Geometry check sheet. Reference: the model listing, model coordinates, mm. A direction names the side the tool comes from. Round coordinates to 2 decimals unless told otherwise and drop trailing zeros. Write each loop counter-clockwise with the first axis right and the second up, starting at its lowest first coordinate (ties: lowest second). Pieces come first, ordered by that corner, then holes. Notation, with made-up numbers: M 87,-8.5 L 111,-8.5 A13 ccw 111,-0.5 Z; hole C 14.5,3.5 d10. An arc over 180 degrees is marked long. Answer in a Markdown table with one row per item. Add a question column.
Autodesk Inventor part; units mm, degrees
ref_plane "YZ Plane" through (0, 0, 0) normal (1, 0, 0) x (0, 1, 0)
ref_plane "XZ Plane" through (0, 0, 0) normal (0, 1, 0) x (-1, 0, 0)
ref_plane "XY Plane" through (0, 0, 0) normal (0, 0, 1) x (1, 0, 0)
sketch "Sketch1" plane through (0, 0, 0) normal (0, 1, 0) x (-1, 0, 0)
  line L0 (-25, -25) -> (25, -25)
  line L1 (25, -25) -> (25, 25)
  line L2 (25, 25) -> (-25, 25)
  line L3 (-25, 25) -> (-25, -25)
  line L4 (-25, -25) -> (25, 25) construction
  line L5 (25, -25) -> (-25, 25) construction
  circle A0 centre (0, 0) radius 2.5
  line L6 (-22.5, -22.5) -> (-27.5, -22.5)
  line L7 (-27.5, -22.5) -> (-27.5, -27.5)
  line L8 (-27.5, -27.5) -> (-22.5, -27.5)
  line L9 (-22.5, -27.5) -> (-22.5, -22.5)
  line L10 (-22.5, -22.5) -> (-27.5, -27.5) construction
  line L11 (-27.5, -22.5) -> (-22.5, -27.5) construction
  line L12 (27.5, -22.5) -> (22.5, -22.5)
  line L13 (22.5, -22.5) -> (22.5, -27.5)
  line L14 (22.5, -27.5) -> (27.5, -27.5)
  line L15 (27.5, -27.5) -> (27.5, -22.5)
  line L16 (27.5, -22.5) -> (22.5, -27.5) construction
  line L17 (22.5, -22.5) -> (27.5, -27.5) construction
  line L18 (27.5, 27.5) -> (22.5, 27.5)
  line L19 (22.5, 27.5) -> (22.5, 22.5)
  line L20 (22.5, 22.5) -> (27.5, 22.5)
  line L21 (27.5, 22.5) -> (27.5, 27.5)
  line L22 (27.5, 27.5) -> (22.5, 22.5) construction
  line L23 (22.5, 27.5) -> (27.5, 22.5) construction
  line L24 (-22.5, 27.5) -> (-27.5, 27.5)
  line L25 (-27.5, 27.5) -> (-27.5, 22.5)
  line L26 (-27.5, 22.5) -> (-22.5, 22.5)
  line L27 (-22.5, 22.5) -> (-22.5, 27.5)
  line L28 (-22.5, 27.5) -> (-27.5, 22.5) construction
  line L29 (-27.5, 27.5) -> (-22.5, 22.5) construction
  circle A1 centre (5, -5) radius 1
  circle A2 centre (5, 5) radius 1
  circle A3 centre (-5, 5) radius 1
  circle A4 centre (-5, -5) radius 1
  point P0 (25, -22.5)
  point P1 (22.5, -25)
  point P2 (-22.5, -25)
  point P3 (-25, -22.5)
  point P4 (-25, 22.5)
  point P5 (-22.5, 25)
  point P6 (22.5, 25)
  point P7 (25, 22.5)
  point P8 (0, -25)
  point P9 (25, 0)
  point P10 (0, 25)
  point P11 (-25, 0)
  dimension "d0" = 50
  dimension "d1" = 50
  dimension "d45" = 5
  dimension "d46" = 5
  dimension "d47" = 5
  dimension "d48" = 5
  dimension "d49" = 5
  dimension "d50" = 5
  dimension "d51" = 5
  dimension "d52" = 5
  dimension "d53" = 5
  dimension "d82" = 2
  dimension "d83" = 2
  dimension "d84" = 2
  dimension "d85" = 2
  dimension "d86" = 5
  dimension "d87" = 5
  dimension "d88" = 5
  dimension "d89" = 5
  dimension "d90" = 5
  dimension "d91" = 5
  dimension "d92" = 5
  dimension "d93" = 5
extrude "Extrusion1" add sketch "Sketch1" along normal blind 5
sketch "Sketch2" plane through (0, 5, 0) normal (0, 1, 0) x (1, 0, 0)
  line L0 (-25, 22.5) -> (-25, -22.5)
  line L1 (-22.5, -25) -> (22.5, -25)
  line L2 (25, -22.5) -> (25, 22.5)
  line L3 (22.5, 25) -> (-22.5, 25)
  line L4 (25, -12.5) -> (20, -12.5)
  line L5 (20, -12.5) -> (20, -7.5)
  line L6 (20, -7.5) -> (25, -7.5)
  line L7 (25, -7.5) -> (25, -12.5)
  line L8 (25, -22.5) -> (25, 22.5)
  line L9 (25, 7.5) -> (20, 7.5)
  line L10 (20, 7.5) -> (20, 12.5)
  line L11 (20, 12.5) -> (25, 12.5)
  line L12 (25, 12.5) -> (25, 7.5)
  line L13 (-25, -12.5) -> (-20, -12.5)
  line L14 (-20, -12.5) -> (-20, -7.5)
  line L15 (-20, -7.5) -> (-25, -7.5)
  line L16 (-25, -7.5) -> (-25, -12.5)
  line L17 (-25, 22.5) -> (-25, -22.5)
  line L18 (-25, 7.5) -> (-20, 7.5)
  line L19 (-20, 7.5) -> (-20, 12.5)
  line L20 (-20, 12.5) -> (-25, 12.5)
  line L21 (-25, 12.5) -> (-25, 7.5)
  line L22 (-22.5, -25) -> (22.5, -25)
  line L23 (-25, 12.5) -> (-20, 12.5)
  line L24 (-20, 12.5) -> (-20, 13.5)
  line L25 (-20, 13.5) -> (-25, 13.5)
  line L26 (-25, 13.5) -> (-25, 12.5)
  line L27 (20, 12.5) -> (25, 12.5)
  line L28 (25, 12.5) -> (25, 13.5)
  line L29 (25, 13.5) -> (20, 13.5)
  line L30 (20, 13.5) -> (20, 12.5)
  line L31 (25, 7.5) -> (20, 7.5)
  line L32 (20, 7.5) -> (20, 6.5)
  line L33 (20, 6.5) -> (25, 6.5)
  line L34 (25, 6.5) -> (25, 7.5)
  line L35 (-20, 7.5) -> (-25, 7.5)
  line L36 (-25, 7.5) -> (-25, 6.5)
  line L37 (-25, 6.5) -> (-20, 6.5)
  line L38 (-20, 6.5) -> (-20, 7.5)
  line L39 (-25, -7.5) -> (-20, -7.5)
  line L40 (-20, -7.5) -> (-20, -6.5)
  line L41 (-20, -6.5) -> (-25, -6.5)
  line L42 (-25, -6.5) -> (-25, -7.5)
  line L43 (-25, -12.5) -> (-20, -12.5)
  line L44 (-20, -12.5) -> (-20, -13.5)
  line L45 (-20, -13.5) -> (-25, -13.5)
  line L46 (-25, -13.5) -> (-25, -12.5)
  line L47 (25, -7.5) -> (20, -7.5)
  line L48 (20, -7.5) -> (20, -6.5)
  line L49 (20, -6.5) -> (25, -6.5)
  line L50 (25, -6.5) -> (25, -7.5)
  line L51 (20, -12.5) -> (25, -12.5)
  line L52 (25, -12.5) -> (25, -13.5)
  line L53 (25, -13.5) -> (20, -13.5)
  line L54 (20, -13.5) -> (20, -12.5)
  line L55 (-25, -22.5) -> (-27.5, -22.5)
  line L56 (-27.5, -22.5) -> (-27.5, -27.5)
  line L57 (-27.5, -27.5) -> (-22.5, -27.5)
  line L58 (-22.5, -27.5) -> (-22.5, -25)
  line L59 (22.5, -25) -> (22.5, -27.5)
  line L60 (22.5, -27.5) -> (27.5, -27.5)
  line L61 (27.5, -27.5) -> (27.5, -22.5)
  line L62 (27.5, -22.5) -> (25, -22.5)
  line L63 (25, 22.5) -> (27.5, 22.5)
  line L64 (27.5, 22.5) -> (27.5, 27.5)
  line L65 (27.5, 27.5) -> (22.5, 27.5)
  line L66 (22.5, 27.5) -> (22.5, 25)
  line L67 (-22.5, 25) -> (-22.5, 27.5)
  line L68 (-22.5, 27.5) -> (-27.5, 27.5)
  line L69 (-27.5, 27.5) -> (-27.5, 22.5)
  line L70 (-27.5, 22.5) -> (-25, 22.5)
  line L71 (-12.5, 25) -> (-7.5, 25)
  line L72 (-7.5, 25) -> (-7.5, 20)
  line L73 (-7.5, 20) -> (-12.5, 20)
  line L74 (-12.5, 20) -> (-12.5, 25)
  line L75 (7.5, 25) -> (12.5, 25)
  line L76 (12.5, 25) -> (12.5, 20)
  line L77 (12.5, 20) -> (7.5, 20)
  line L78 (7.5, 20) -> (7.5, 25)
  line L79 (-12.5, -25) -> (-7.5, -25)
  line L80 (-7.5, -25) -> (-7.5, -20)
  line L81 (-7.5, -20) -> (-12.5, -20)
  line L82 (-12.5, -20) -> (-12.5, -25)
  line L83 (7.5, -25) -> (12.5, -25)
  line L84 (12.5, -25) -> (12.5, -20)
  line L85 (12.5, -20) -> (7.5, -20)
  line L86 (7.5, -20) -> (7.5, -25)
  line L87 (22.5, 25) -> (-22.5, 25)
  line L88 (-12.5, -20) -> (-13.5, -20)
  line L89 (-13.5, -20) -> (-13.5, -25)
  line L90 (-13.5, -25) -> (-12.5, -25)
  line L91 (-12.5, -25) -> (-12.5, -20)
  line L92 (-7.5, -20) -> (-6.5, -20)
  line L93 (-6.5, -20) -> (-6.5, -25)
  line L94 (-6.5, -25) -> (-7.5, -25)
  line L95 (-7.5, -25) -> (-7.5, -20)
  line L96 (7.5, -20) -> (6.5, -20)
  line L97 (6.5, -20) -> (6.5, -25)
  line L98 (6.5, -25) -> (7.5, -25)
  line L99 (7.5, -25) -> (7.5, -20)
  line L100 (12.5, -20) -> (13.5, -20)
  line L101 (13.5, -20) -> (13.5, -25)
  line L102 (13.5, -25) -> (12.5, -25)
  line L103 (12.5, -25) -> (12.5, -20)
  line L104 (-7.5, 25) -> (-6.5, 25)
  line L105 (-6.5, 25) -> (-6.5, 20)
  line L106 (-6.5, 20) -> (-7.5, 20)
  line L107 (-7.5, 20) -> (-7.5, 25)
  line L108 (7.5, 25) -> (6.5, 25)
  line L109 (6.5, 25) -> (6.5, 20)
  line L110 (6.5, 20) -> (7.5, 20)
  line L111 (7.5, 20) -> (7.5, 25)
  line L112 (12.5, 25) -> (13.5, 25)
  line L113 (13.5, 25) -> (13.5, 20)
  line L114 (13.5, 20) -> (12.5, 20)
  line L115 (12.5, 20) -> (12.5, 25)
  line L116 (-12.5, 25) -> (-13.5, 25)
  line L117 (-13.5, 25) -> (-13.5, 20)
  line L118 (-13.5, 20) -> (-12.5, 20)
  line L119 (-12.5, 20) -> (-12.5, 25)
  point P0 (0, 0)
  point P1 (-25, 25)
  point P2 (-25, -25)
  point P3 (25, -25)
  point P4 (25, 25)
  point P5 (20, -10)
  point P6 (20, 10)
  point P7 (-25, 10)
  point P8 (-25, -10)
  point P9 (-25, 6.5)
  point P10 (-25, 13.5)
  point P11 (25, 13.5)
  point P12 (25, 6.5)
  point P13 (25, -13.5)
  point P14 (-25, -13.5)
  point P15 (25, 10)
  point P16 (-25, 0)
  point P17 (0, -25)
  point P18 (-10, -25)
  point P19 (10, -25)
  point P20 (0, 25)
  point P21 (10, 25)
  point P22 (-10, 25)
  point P23 (0, 25)
  dimension "d9" = 5
  dimension "d10" = 5
  dimension "d11" = 5
  dimension "d12" = 5
  dimension "d13" = 5
  dimension "d14" = 5
  dimension "d15" = 5
  dimension "d16" = 5
  dimension "d21" = 5
  dimension "d22" = 1
  dimension "d23" = 5
  dimension "d24" = 1
  dimension "d25" = 5
  dimension "d26" = 1
  dimension "d27" = 5
  dimension "d28" = 1
  dimension "d29" = 5
  dimension "d30" = 1
  dimension "d31" = 5
  dimension "d32" = 1
  dimension "d33" = 5
  dimension "d34" = 1
  dimension "d35" = 5
  dimension "d36" = 1
  dimension "d43" = 10
  dimension "d54" = 5
  dimension "d55" = 5
  dimension "d56" = 5
  dimension "d57" = 5
  dimension "d58" = 5
  dimension "d59" = 5
  dimension "d60" = 5
  dimension "d61" = 5
  dimension "d62" = 10
  dimension "d63" = 10
  dimension "d64" = 10
  dimension "d65" = 10
  dimension "d66" = 1
  dimension "d67" = 5
  dimension "d68" = 1
  dimension "d69" = 5
  dimension "d70" = 1
  dimension "d71" = 5
  dimension "d72" = 1
  dimension "d73" = 5
  dimension "d74" = 1
  dimension "d75" = 5
  dimension "d76" = 1
  dimension "d77" = 5
  dimension "d78" = 1
  dimension "d79" = 5
  dimension "d80" = 1
  dimension "d81" = 5
extrude "Extrusion2" add sketch "Sketch2" along normal blind 5 contours L25 L24 L20 L0 | L18 L38 L37 L0 | L41 L40 L15 L0 | L3 L74 L118 L117 | L13 L44 L45 L0 | L3 L105 L106 L72 | L3 L78 L110 L109 | L3 L113 L114 L76 | L89 L88 L82 L1 | L80 L92 L93 L1 | L97 L96 L86 L1 | L2 L11 L30 L29 | L84 L100 L101 L1 | L2 L33 L32 L9 | L2 L6 L48 L49 | L2 L53 L54 L4
equation "\"BendRadius\" = Thickness"
equation "\"BendReliefWidth\" = Thickness"
equation "\"BendReliefDepth\" = 0.5 * Thickness"
equation "\"CornerReliefSize\" = 4 * Thickness"
equation "\"MinimumRemnant\" = 2 * Thickness"
equation "\"TransitionRadius\" = BendRadius"
equation "\"JacobiRadiusSize\" = BendRadius"
equation "\"GapSize\" = Thickness"
properties part number "base"
Item 1: Gauge pin test, flat ends, axial feed: pin 1 Ø5 at (y, z) = (1.5, 1) entering from +X; pin 2 Ø1 at (x, z) = (-21.5, -21.5) entering from +Y; pin 3 Ø0.8 at (x, y) = (7, 7.5) entering from +Z. Record the tip position at first contact, or that the pin passes through.
Item 2: Section check C-C, the plane y = 1.5. Record the boundary of the cut face in (x, z).
Item 3: Section check B-B, the plane x = 5. Record the boundary of the cut face in (y, z).
Item 4: Section check D-D, the plane x = -0.5. Record the boundary of the cut face in (y, z).
Item 5: Mould release check, pull along Z, two halves, no side actions. Record for faces 1 (the flat face through (23, 7, 12.5)), 2 (the flat face through (-22, 7, -13.5)), 3 (the flat face through (-6.5, 7, -23)): +Z half, -Z half, draft (parallel to the pull), parting line (faces both ways), or undercut.
Item 6: Scan lines: probe 1 along Z at (x, y) = (5, 2.75); probe 2 along X at (y, z) = (6.5, -23.5); probe 3 along X at (y, z) = (3, -17.5). Record each from-to range of solid material in increasing order. Write a range as from..to.
Item 7: Access from +Z, -Z, +X, -X, +Y, -Y to the whole of each face (thin tool, end or side, straight path). Record for faces 4 (the flat face through (-7.5, 7, 23)), 5 (the flat face through (13.5, 7, 22)), 6 (the flat face through (-26, 2, 22.5)), 7 (the flat face through (26, 2, -22.5)), 8 (the flat face through (-22, 7, -12.5)).
Item 8: Section check A-A, the plane z = -5. Record the boundary of the cut face in (x, y).
Result sheet:
| question | item | result |
|---|---|---|
| 1 | pin 1 | stops at x = 25 |
| 1 | pin 2 | stops at y = 5 |
| 1 | pin 3 | stops at z = 25 |
| 2 | outline | M -27.5,-27.5 L -22.5,-27.5 L -22.5,-25 L 22.5,-25 L 22.5,-27.5 L 27.5,-27.5 L 27.5,-22.5 L 25,-22.5 L 25,22.5 L 27.5,22.5 L 27.5,27.5 L 22.5,27.5 L 22.5,25 L -22.5,25 L -22.5,27.5 L -27.5,27.5 L -27.5,22.5 L -25,22.5 L -25,-22.5 L -27.5,-22.5 Z; hole C -5,-5 d2; hole C -5,5 d2; hole C 0,0 d5; hole C 5,-5 d2; hole C 5,5 d2 |
| 3 | outline | M 0,-25 L 5,-25 L 5,-6 L 0,-6 Z; M 0,-4 L 5,-4 L 5,4 L 0,4 Z; M 0,6 L 5,6 L 5,25 L 0,25 Z |
| 4 | outline | M 0,-25 L 5,-25 L 5,-2.45 L 0,-2.45 Z; M 0,2.45 L 5,2.45 L 5,25 L 0,25 Z |
| 5 | face 1 | undercut |
| 5 | face 2 | -Z half |
| 5 | face 3 | draft |
| 6 | probe 1 | z = -25..-6, -4..4, 6..25 |
| 6 | probe 2 | x = -13.5..-12.5, -7.5..-6.5, 6.5..7.5, 12.5..13.5 |
| 6 | probe 3 | x = -25..25 |
| 7 | face 4 | +Z, -Z, +Y |
| 7 | face 5 | +Z, -Z, +X, +Y |
| 7 | face 6 | -X, +Y, -Y |
| 7 | face 7 | +X, +Y, -Y |
| 7 | face 8 | +X, -X, +Y |
| 8 | outline | M -25,0 L -6,0 L -6,5 L -25,5 Z; M -4,0 L 4,0 L 4,5 L -4,5 Z; M 6,0 L 25,0 L 25,5 L 6,5 Z |
